```python
from build123d import *

# Parameters (mm, degrees)
F3_DEPTH = 2.5
F4_W     = 9.8994949366
F4_H     = 9.8994949366
F5_DEPTH = 2.001


with BuildPart() as f1:
    # F0 (on Front) → F1 (revolve)
    with BuildSketch(Plane.XZ):
        Polygon((-23.5, 0), (0, 0), (0, 2), (-11.79, 2), (-11.79, 13), (-11.79, 15.5), (-12.79, 15.5), (-12.79, 13), (-13.79, 13), (-13.79, 2), (-23.5, 2), align=None)
    revolve(axis=Axis((0, 0, 1), (0, 0, 1)))

    # F2 (on face) → F3 (cut, through all)
    with BuildSketch(Plane.XY.offset(15.5)):
        with BuildLine():
            Line((-11.7476165971, 0.9988014258), (-12.7440217368, 1.0835174076))
            ThreePointArc((-12.7440217368, 1.0835174076), (-12.79, 0), (-12.7440217368, -1.0835174076))
            Line((-12.7440217368, -1.0835174076), (-11.7476165971, -0.9988014258))
            ThreePointArc((-11.7476165971, -0.9988014258), (-11.79, 0), (-11.7476165971, 0.9988014258))
        make_face()
        with BuildLine():
            ThreePointArc((12.7440217368, -1.0835174076), (12.7785002644, -0.5422462479), (12.79, 0))
            ThreePointArc((12.79, 0), (12.7785002644, 0.5422462479), (12.7440217368, 1.0835174076))
            Line((12.7440217368, 1.0835174076), (11.7476165971, 0.9988014258))
            ThreePointArc((11.7476165971, 0.9988014258), (11.7793993837, 0.4998501378), (11.79, 0))
            ThreePointArc((11.79, 0), (11.7793993837, -0.4998501378), (11.7476165971, -0.9988014258))
            Line((11.7476165971, -0.9988014258), (12.7440217368, -1.0835174076))
        make_face()
    extrude(amount=-F3_DEPTH, mode=Mode.SUBTRACT)

    # F4 (on face) → F5 (cut, through all)
    with BuildSketch(Plane.XY.offset(2)):
        Rectangle(F4_W, F4_H)
    extrude(amount=-F5_DEPTH, mode=Mode.SUBTRACT)


solid = f1.part
```
Input: part model. Units: mm. Frame: model coordinates. A direction names the side the tool comes from. Give positions to 0.01 mm unless a question says otherwise; leave off trailing zeros. Loops run counter-clockwise (first coordinate to the right, second up) from the corner with the lowest first, then second, coordinate; pieces in that order, holes last. Notation, with made-up numbers: M -10.75,-34.5 L 23.25,-34.5 A15 ccw 23.25,-28.5 Z; hole C 11.25,86.25 d9. An arc over 180 degrees is marked long. Answer as CSV lines item,"result". Start each with the question number.
1. Section D-D on x = 17. Return loops of the section in (y, z), plus the area to 3 significant figures.
2. Section C-C on z = 6.5. Return loops of the section in (x, y).
3. Line query: L1, parallel to X at y = 0, z = 7.5; L2, parallel to Z at x = -9, y = -7. Output: solid intervals per line, ascending.
4. Pull-direction query (X, two-part tool) for faces 6 (the face through (-0.266, -12.787, 14.232)), 7 (the face through (-2, 12, 15.5)), 8 (the face through (5.1, -0.2, 2)); classes: released by +X, released by -X, zero draft, split by the parting line, or undercut.
5. Reachability of faces 1 (the face through (0.266, 12.787, 14.232)), 2 (the face through (4.95, 0, 1)), 3 (the face through (12, 0, 13)), 4 (the face through (0, -12, 15.5)), 5 (the face through (0, -6, 0)) from +Z, -Z, +X, -X, +Y, -Y: full face, straight path, thin tool, end or side. Return the list, or none.
6. Section A-A on y = 0. Return loops of the section in (x, z).
7. Section B-B on x = 0. Return loops of the section in (y, z), plus the area to 3 significant figures.
8. Pin query (flat end, axial travel): P1, Ø1, axis at x = 2.5, y = 10.5, coming from the -Z side; P2, Ø21, axis at x = 0, y = 0, coming from the +Z side; P3, Ø4, axis at y = -7, z = 7.5, coming from the +X side; P4, Ø1.6, axis at y = 2, z = 1, coming from the -X side. Return the tip coordinate at first contact, or that it passes through.
Computed values:
1,outline,"M -16.22,0 L 16.22,0 L 16.22,2 L -16.22,2 Z"
1,area,"64.9 mm²"
2,outline,"C 0,0 d27.58; hole C 0,0 d23.58"
3,L1,"x = -13.79 to -11.79, 11.79 to 13.79"
3,L2,"z = 0 to 2"
4,face 6,"split by the parting line"
4,face 7,"zero draft"
4,face 8,"undercut"
5,face 1,"+Z, +Y"
5,face 2,"+Z, -Z"
5,face 3,"+Z"
5,face 4,"+Z, +X, -X, +Y, -Y"
5,face 5,"-Z, +X, -X, +Y, -Y"
6,outline,"M -23.5,0 L -4.95,0 L -4.95,2 L -11.79,2 L -11.79,13 L -13.79,13 L -13.79,2 L -23.5,2 Z; M 4.95,0 L 23.5,0 L 23.5,2 L 13.79,2 L 13.79,13 L 11.79,13 L 11.79,2 L 4.95,2 Z"
7,outline,"M -23.5,0 L -4.95,0 L -4.95,2 L -11.79,2 L -11.79,15.5 L -12.79,15.5 L -12.79,13 L -13.79,13 L -13.79,2 L -23.5,2 Z; M 4.95,0 L 23.5,0 L 23.5,2 L 13.79,2 L 13.79,13 L 12.79,13 L 12.79,15.5 L 11.79,15.5 L 11.79,2 L 4.95,2 Z"
7,area,"123 mm²"
8,P1,"stops at z = 0"
8,P2,"stops at z = 2"
8,P3,"stops at x = 12.85"
8,P4,"stops at x = -23.47"
